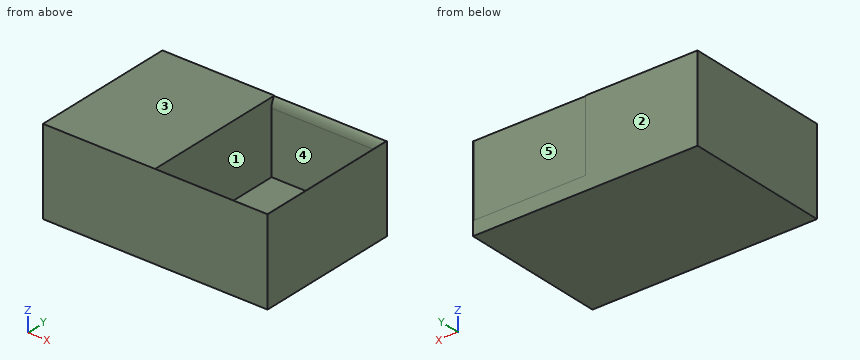
from build123d import *

# Parameters (mm, degrees)
F1_DEPTH      = 25.4
F1_DEPTH_BACK = 32.512
F3_DEPTH      = 39.37
F3_DEPTH_BACK = 23.114
F6_START      = -47.498
F5_W          = 76.2000009418
F5_H          = 48.3009684831
F6_DEPTH      = 2.286
F7_T1_DEPTH   = 76.1999934912


# Not quite as in the source:
# - a fillet or chamfer that OpenCascade refuses, or shapes differently, is made with other operations: its cross-section is extruded or revolved along the edge and cut away or added


with BuildPart() as f1:
    # F0 (on Top) → F1 (new body, two sides)
    with BuildSketch(Plane.XY) as f1_sk:
        Polygon((0, 0), (0, -50), (76.3228982687, -50), (76.3228982687, 50), (0, 50), align=None)
        Polygon((-75.9541913867, -50), (0, -50), (0, 0), (0, 50), (-75.9541913867, 50), align=None)
    extrude(amount=F1_DEPTH)
    extrude(f1_sk.sketch, amount=-F1_DEPTH_BACK)


with BuildPart() as f3:
    # F2 (on Top) → F3 (new body, two sides)
    with BuildSketch(Plane.XY) as f3_sk:
        Polygon((0, 50.1445159316), (0, 0), (0, -49.9601624906), (76.1999934912, -49.9601624906), (76.1999934912, 50.1445159316), align=None)
    extrude(amount=F3_DEPTH)
    extrude(f3_sk.sketch, amount=-F3_DEPTH_BACK)


with BuildPart() as f1_1:
    add(f1.part)

    # F4: cut F3
    add(f3.part, mode=Mode.SUBTRACT)

    # F5 (on Front) → F6 (join)
    with BuildSketch(Plane.XZ.offset(F6_START)):
        with Locations((38.1000004709, 1.1061290279)):
            Rectangle(F5_W, F5_H)
    extrude(amount=-F6_DEPTH)

    # F7: fillet of radius 10 on 1 edges, made by hand

    # F7_s2 → F7_t1 (cut)
    with BuildSketch(Plane.YZ):
        with BuildLine():
            ThreePointArc((47.498, 18.8931076318), (48.0868364163, 22.2739359327), (49.784, 25.2566132694))
            Line((49.784, 25.2566132694), (47.498, 25.2566132694))
            Line((47.498, 25.2566132694), (47.498, 18.8931076318))
        make_face()
    extrude(amount=F7_T1_DEPTH, mode=Mode.SUBTRACT)


solid = f1_1.part
Verification items for the finished model (mm, model axes). Face numbers are marked on the shaded views. A direction names the side the tool comes from. Give positions to 0.01 mm unless a question says otherwise; leave off trailing zeros. Write each loop counter-clockwise with the first axis right and the second up, starting at its lowest first coordinate (ties: lowest second). Pieces come first, ordered by that corner, then holes.
(1) Cross-section at D-D (z = 21). Enter the section's corners in (x, y), plus the area to 3 significant figures.
(2) Cross-section at A-A (z = 2). Enter the section's corners in (x, y).
(3) Cross-section at C-C (y = -37.5). Enter the section's corners in (x, z), plus the area to 3 significant figures.
(4) Mould release check, pull along Y, two halves, no side actions. Record for the marked faces 3, 4 and 5: +Y half, -Y half, draft (parallel to the pull), parting line (faces both ways), or undercut.
(5) Material ranges on line 1 (Z direction, x = 9.5, y = 33.5), recorded low to high.
(6) Access from +Z, -Z, +X, -X, +Y, -Y to the whole of each face (thin tool, end or side, straight path). Record for the marked faces 1 and 2.
(7) Gauge pin test, flat end, axial feed: pin 1 (10 mm diameter, centred on x = 12.5, y = 5.5, fed in from +Z). Record the tip position at first contact, or that the pin passes through.
Worked out:
1. outline: (-75.95, -50) - (76.32, -50) - (76.32, 50) - (76.2, 50) - (76.2, 49.78) - (0, 49.78) - (0, 50) - (-75.95, 50) - close; hole (0, -49.96) - (76.2, -49.96) - (76.2, 47.72) - (0, 47.72) - close
1. area: 7,770 mm2
2. outline: (-75.95, -50) - (76.32, -50) - (76.32, 50) - (76.2, 50) - (76.2, 49.78) - (0, 49.78) - (0, 50) - (-75.95, 50) - close; hole (0, -49.96) - (76.2, -49.96) - (76.2, 47.5) - (0, 47.5) - close
3. outline: (-75.95, -32.51) - (76.32, -32.51) - (76.32, 25.4) - (76.2, 25.4) - (76.2, -23.11) - (0, -23.11) - (0, 25.4) - (-75.95, 25.4) - close
3. area: 5,120 mm2
4. face 3: draft
4. face 4: undercut
4. face 5: +Y half
5. line 1: z = -32.51 to -23.11
6. face 1: +Z
6. face 2: +Z, -Z, +X, -X, +Y
7. pin 1: stops at z = -23.11
